from build123d import *

# Parameters (mm, degrees)
PAD_DEPTH = 1


with BuildPart() as part:
    # Sketch → Pad (new body)
    with BuildSketch(Plane.XZ):
        Polygon((450, 0), (318.198052, 318.198052), (0, 450), (-318.198052, 318.198052), (-450, 0), (-318.198052, -318.198052), (0, -450), (318.198052, -318.198052), align=None)
    extrude(amount=PAD_DEPTH)


solid = part.part
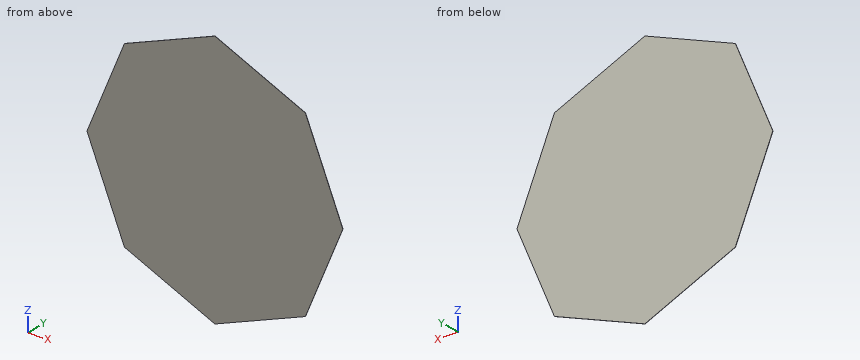
Source: CAD feature listing. Evaluate the final solid. Frame: model axes, mm. Give positions to 0.01 mm unless a question says otherwise; leave off trailing zeros. Write each loop counter-clockwise with the first axis right and the second up, starting at its lowest first coordinate (ties: lowest second). Pieces come first, ordered by that corner, then holes. Notation, with made-up numbers: M -33.75,46 L -16.75,46 A13 ccw -16.75,63 Z; hole C 26,39 d11. An arc over 180 degrees is marked long. Return JSON: item names as keys, results as strings. Group by question number.
1) Cut plane C-C, the plane z = -222. Output: boundary loops of the cut face in (x, y).
2) Cut plane A-A, the plane y = -0.85. Output: boundary loops of the cut face in (x, z).
3) Material intervals for line 1 along Z through (x, y) = (55.5, -0.15); line 2 along Z through (x, y) = (188, -0.05); line 3 along X through (y, z) = (-0.15, -308.5), sorted ascending. Write a range as [from, to].
4) Cut plane B-B, the plane x = -260.5. Output: boundary loops of the cut face in (y, z), plus the area to 3 significant figures.
Recorded:
{
 "1": {"outline": "M -358.04,-1 L 358.04,-1 L 358.04,0 L -358.04,0 Z"},
 "2": {"outline": "M -450,0 L -318.2,-318.2 L 0,-450 L 318.2,-318.2 L 450,0 L 318.2,318.2 L 0,450 L -318.2,318.2 Z"},
 "3": {"line 1": "z = [-427.01, 427.01]", "line 2": "z = [-372.13, 372.13]", "line 3": "x = [-322.22, 322.22]"},
 "4": {"outline": "M -1,-342.1 L 0,-342.1 L 0,342.1 L -1,342.1 Z", "area": "684 mm²"}
}
